Could you check a few things on this model? Use its own coordinates, in mm. Face numbers are marked on the shaded views. A direction names the side the tool comes from. Round coordinates to 2 decimals unless told otherwise and drop trailing zeros. Loops run counter-clockwise (first coordinate to the right, second up) from the corner with the lowest first, then second, coordinate; pieces in that order, holes last. Notation, with made-up numbers: (78, 42) -> (104, 42) arc R27 cw to (104, 74) -> close; hole circle Ø11 at (1.25, -40). An arc over 180 degrees is marked (long way). One line per item, written item: value.
Autodesk Inventor part; units mm, degrees
ref_plane "YZ Plane" through (0, 0, 0) normal (1, 0, 0) x (0, 1, 0)
ref_plane "XZ Plane" through (0, 0, 0) normal (0, 1, 0) x (-1, 0, 0)
ref_plane "XY Plane" through (0, 0, 0) normal (0, 0, 1) x (1, 0, 0)
sketch "Sketch1" plane through (0, 0, 0) normal (0, 0, 1) x (1, 0, 0)
  line L0 (0, 38.5) -> (0, -38.5) construction
  line L1 (-38.5, 0) -> (38.5, 0) construction
  line L2 (-27.5, 27.5) -> (27.5, 27.5)
  line L3 (27.5, 27.5) -> (27.5, -27.5)
  line L4 (27.5, -27.5) -> (-27.5, -27.5)
  line L5 (-27.5, -27.5) -> (-27.5, 27.5)
  point P0 (0, 0)
  dimension "d0" = 55
  dimension "d1" = 55
extrude "Extrusion1" add sketch "Sketch1" along normal blind 20
sketch "Sketch4" plane through (0, 0, 20) normal (0, 0, 1) x (1, 0, 0)
  line L0 (-38.5, 0) -> (38.5, 0) construction
  line L1 (0, 38.5) -> (0, -38.5) construction
  line L2 (-22.6, 22.6) -> (22.6, 22.6) construction
  line L3 (22.6, 22.6) -> (22.6, -22.6) construction
  line L4 (22.6, -22.6) -> (-22.6, -22.6) construction
  line L5 (-22.6, -22.6) -> (-22.6, 22.6) construction
  point P0 (0, 0)
  dimension "d15" = 45.2
  dimension "d16" = 45.2
hole "Hole2" at (-22.6, 22.6, 20) at (22.6, 22.6, 20) at (22.6, -22.6, 20) at (-22.6, -22.6, 20) at (-22.6, 22.6, 20) at (22.6, 22.6, 20) direction (0, 0, -1) diameter 5 depth 8
sketch "Sketch5" plane through (0, 0, 20) normal (0, 0, 1) x (1, 0, 0)
  circle A0 centre (-22.6, 22.6) radius 2.5
  circle A1 centre (22.6, -22.6) radius 2.5
  line L0 (-22.6, 22.6) -> (22.6, 22.6)
  line L1 (22.6, 22.6) -> (22.6, -22.6)
  line L2 (22.6, -22.6) -> (-22.6, -22.6)
  line L3 (-22.6, -22.6) -> (-22.6, 22.6)
  point P0 (0, 0)
extrude "Extrusion3" cut sketch "Sketch5" against normal blind 8 contours L0 L1 A1 L2 L3 A0 | A0 L3 L0 | L1 L2 A1 picked at (-20.9542, 22.4146) picked at (21.1977, -21.7189)
sketch "Sketch6" plane through (-27.5, -27.5, 0) normal (-1, 0, 0) x (0, 0, 1)
  line L0 (0, 55) -> (20, 55)
  line L1 (0, 0) -> (20, 0)
  line L2 (20, 7.4) -> (12, 7.4) construction
  line L3 (20, 47.6) -> (20, 7.4) construction
  line L4 (12, 47.6) -> (20, 47.6) construction
  line L5 (12, 7.4) -> (12, 47.6) construction
  line L6 (16, 47.6) -> (16, 7.4) construction
  point P0 (0, 27.5)
  point P1 (16, 40)
  point P2 (16, 15)
  dimension "d26" = 15
  dimension "d27" = 15
hole "Hole3" at (-27.5, 12.5, 16) at (-27.5, -12.5, 16) direction (1, 0, 0) diameter 3.242 end up to surface
sketch "Sketch8" plane through (0, 0, 0) normal (0, 0, -1) x (-1, 0, 0)
  line L0 (27.5, 27.5) -> (-27.5, 27.5) construction
  line L1 (-27.5, 27.5) -> (-27.5, -27.5) construction
  line L2 (-27.5, -27.5) -> (27.5, -27.5) construction
  line L3 (27.5, -27.5) -> (27.5, 27.5) construction
  line L4 (0, -38.5) -> (0, 38.5) construction
  line L5 (-38.5, 0) -> (38.5, 0) construction
  line L6 (-12.5, -12.5) -> (12.5, -12.5)
  line L7 (12.5, -12.5) -> (12.5, 12.5)
  line L8 (12.5, 12.5) -> (-12.5, 12.5)
  line L9 (-12.5, 12.5) -> (-12.5, -12.5)
  point P0 (0, 0)
  dimension "d44" = 25
  dimension "d45" = 25
extrude "Extrusion4" cut sketch "Sketch8" against normal blind 6
sketch "Sketch9" plane through (0, 0, 0) normal (0, 0, -1) x (-1, 0, 0)
  line L0 (12.5, 12.5) -> (12.5, -12.5) construction
  line L1 (12.5, -12.5) -> (-12.5, -12.5) construction
  line L2 (-12.5, -12.5) -> (-12.5, 12.5) construction
  line L3 (-12.5, 12.5) -> (12.5, 12.5) construction
  line L4 (27.5, 27.5) -> (-27.5, 27.5) construction
  line L5 (-27.5, 27.5) -> (-27.5, -27.5) construction
  line L6 (-27.5, -27.5) -> (27.5, -27.5) construction
  line L7 (27.5, -27.5) -> (27.5, 27.5) construction
  line L8 (12.5, -12.5) -> (-12.5, -12.5) construction
  point P0 (0, 0)
hole "Hole5" at (-12.5, 12.5, 0) at (-12.5, -12.5, 0) at (12.5, -12.5, 0) at (12.5, 12.5, 0) direction (0, 0, 1) diameter 3 depth 6
sketch "Sketch10" plane through (0, 0, 6) normal (0, 0, -1) x (-1, 0, 0)
  point P0 (0, 0)
  point P1 (0, 0)
hole "Hole6" at (0, 0, 6) direction (0, 0, 1) diameter 3.242 depth 4 tip angle 118
ref_plane "SplitPLane" through (0, 0, 6) normal (0, 0, -1) x (-1, 0, 0)
split "Split2" plane through (0, 0, 6) removes the side toward (0, 0, -1)
properties part number "Large-cuvette-mount-40mm-V4_top_extra0.2mm" material "PC/ABS Plastic"
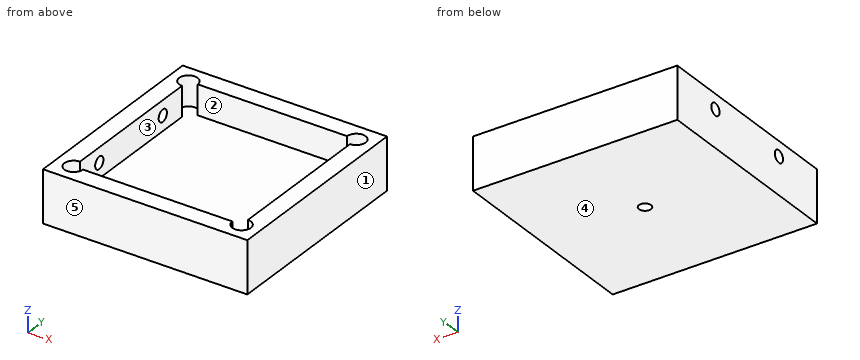
(1) For the marked faces 1 and 2, which set-ups out of +Z, -Z, +X, -X, +Y, -Y let a thin tool reach every point of the face, with its end or its side?
Recorded:
face 1: +Z, -Z, +X, +Y, -Y
face 2: +Z
(2) If I drill on L1, parallel to X at y = -5, z = 17.75; L2, parallel to X at y = 23.5, z = 14.5, over which ranges is the centre line in solid material (lowest first)?
Recorded:
L1: -27.5 to -22.6, 22.6 to 27.5
L2: -27.5 to -24.93, -20.27 to 20.27, 24.93 to 27.5
(3) Thinking about a two-plate mould opening in Y: for the marked faces 3, 4 and 5, which applies, released by +Y, released by -Y, zero draft, split by the parting line, or undercut?
Recorded:
face 3: undercut
face 4: zero draft
face 5: released by -Y
(4) If we section it at A-A, the plane z = 13: Please give me the cut outline in (x, y).
Recorded:
outline: (-27.5, -27.5) -> (27.5, -27.5) -> (27.5, 27.5) -> (-27.5, 27.5) -> close; hole (-22.6, -20.1) arc R2.5 ccw (long way) to (-20.1, -22.6) -> (20.1, -22.6) arc R2.5 ccw (long way) to (22.6, -20.1) -> (22.6, 20.1) arc R2.5 ccw (long way) to (20.1, 22.6) -> (-20.1, 22.6) arc R2.5 ccw (long way) to (-22.6, 20.1) -> close
(5) If we section it at D-D, the plane x = 9.5: Please give me the cut outline in (y, z).
Recorded:
outline: (-27.5, 6) -> (27.5, 6) -> (27.5, 20) -> (22.6, 20) -> (22.6, 12) -> (-22.6, 12) -> (-22.6, 20) -> (-27.5, 20) -> close
(6) If we section it at B-B, the plane y = -12.5: Please give me the cut outline in (x, z), then the cut area to 3 significant figures.
Recorded:
outline: (-27.5, 6) -> (27.5, 6) -> (27.5, 20) -> (22.6, 20) -> (22.6, 12) -> (-22.6, 12) -> (-22.6, 14.38) -> (-27.5, 14.38) -> close; (-27.5, 17.62) -> (-22.6, 17.62) -> (-22.6, 20) -> (-27.5, 20) -> close
area: 393 mm²
(7) If we section it at C-C, the plane z = 16: Please give me the cut outline in (x, y).
Recorded:
outline: (-27.5, -27.5) -> (27.5, -27.5) -> (27.5, 27.5) -> (-27.5, 27.5) -> (-27.5, 14.12) -> (-22.6, 14.12) -> (-22.6, 20.1) arc R2.5 cw (long way) to (-20.1, 22.6) -> (20.1, 22.6) arc R2.5 cw (long way) to (22.6, 20.1) -> (22.6, -20.1) arc R2.5 cw (long way) to (20.1, -22.6) -> (-20.1, -22.6) arc R2.5 cw (long way) to (-22.6, -20.1) -> (-22.6, -14.12) -> (-27.5, -14.12) -> close; (-27.5, -10.88) -> (-22.6, -10.88) -> (-22.6, 10.88) -> (-27.5, 10.88) -> close
